from build123d import *

# Parameters (mm, degrees)
SKETCH8_R           = 12.426789642
BOSS_EXTRUDE3_DEPTH = 8.89
BOSS_EXTRUDE3_TAPER = 15
SKETCH9_R           = 9.553107684
CUT_EXTRUDE1_DEPTH  = 0.508
CUT_EXTRUDE4_REACH  = 23.683


with BuildPart() as part:
    # Sketch7 → Revolve1 (revolve)
    with BuildSketch(Plane.XY, mode=Mode.PRIVATE) as revolve1_sk:
        Polygon((9.553107684, 0), (5.743107684, 3.81), (8.616789642, 3.81), (12.426789642, 0), align=None)
    revolve(revolve1_sk.sketch.rotate(Axis((0, 0, 0), (0, 1, 0)), 90), axis=Axis((0, 0, 0), (0, 1, 0)))

    # Sketch8 → Boss-Extrude3 (add)
    with BuildSketch(Plane.XZ):
        Circle(SKETCH8_R)
    extrude(amount=BOSS_EXTRUDE3_DEPTH, taper=BOSS_EXTRUDE3_TAPER)

    # Sketch9 → Cut-Extrude1 (cut)
    with BuildSketch(Plane(origin=(0, 0, 0), x_dir=(1, 0, 0), z_dir=(0, 1, 0))):
        with Locations(Location((0, 0, 0), (0, 0, 270))):
            Circle(SKETCH9_R)
    extrude(amount=-CUT_EXTRUDE1_DEPTH, mode=Mode.SUBTRACT)

    # Cut-Extrude4: up to this face of the body (flat: up to its plane)
    cut_extrude4_end = Plane(part.part.faces().sort_by_distance((0, -0.508, 0))[0])
    # Sketch13 → Cut-Extrude4 (cut, up to the picked face)
    with BuildSketch(Plane(origin=(0, 3.81, 0), x_dir=(1, 0, 0), z_dir=(0, 1, 0)), mode=Mode.PRIVATE) as cut_extrude4_sk1:
        with BuildLine():
            Line((-5.743107684, 0), (-8.89978102, 8.672888712))
            ThreePointArc((-8.89978102, 8.672888712), (0, 12.426789642), (8.89978102, 8.672888712))
            Line((8.89978102, 8.672888712), (5.743107684, 0))
            ThreePointArc((5.743107684, 0), (0, 5.743107684), (-5.743107684, 0))
        make_face()
    cut_extrude4_tool1 = split(extrude(cut_extrude4_sk1.sketch, amount=-CUT_EXTRUDE4_REACH, mode=Mode.PRIVATE), bisect_by=cut_extrude4_end, keep=Keep.BOTH, mode=Mode.PRIVATE)
    add(cut_extrude4_tool1.solids().sort_by(Axis((0, 3.81, -7.700849), (0, -1, 0)))[0], mode=Mode.SUBTRACT)


solid = part.part
Can you work these out from the model? Positions are in its coordinate system, mm. A direction names the side the tool comes from. Round coordinates to 2 decimals unless told otherwise and drop trailing zeros. Write each loop counter-clockwise with the first axis right and the second up, starting at its lowest first coordinate (ties: lowest second). Pieces come first, ordered by that corner, then holes. Notation, with made-up numbers: M 86.5,38.5 L 141.5,38.5 A27 ccw 141.5,71.5 Z; hole C 5.5,-12.75 d10. An arc over 180 degrees is marked long. Use a Markdown table: item, result.
Item 1: I want a section at B-B (y = -5). List the corners of the cut face in (x, z) for me, and give its area (3 significant figures).
Found:
| item | result |
|---|---|
| outline | C 0,0 d22.17 |
| area | 386 mm2 |
Item 2: I want a section at D-D (y = 1). List the corners of the cut face in (x, z) for me.
Found:
| item | result |
|---|---|
| outline | M -8.52,-7.62 L -7.34,-4.39 A8.55 cw long 7.34,-4.39 L 8.52,-7.62 A11.43 ccw long Z |
Item 3: If I drill on line 1 along Y through (x, z) = (-3.75, -1.25); line 2 along Y through (x, z) = (6.75, 6.5); line 3 along X through (y, z) = (-0.15, 0), over which ranges is the centre line in solid material (lowest first)? Write a range as [from, to].
Found:
| item | result |
|---|---|
| line 1 | y = [-8.89, -0.51] |
| line 2 | y = [-8.89, -0.51], [0.18, 3.06] |
| line 3 | x = [-12.39, -9.55], [9.55, 12.39] |
Item 4: I want a section at A-A (x = 0). List the corners of the cut face in (y, z) for me.
Found:
| item | result |
|---|---|
| outline | M -8.89,-10.04 L -0.51,-12.29 L -0.51,9.55 L 0,9.55 L 3.81,5.74 L 3.81,8.62 L 0,12.43 L -8.89,10.04 Z |
Item 5: We'd pull the mould along Z, two halves only. Please class faces 3 (the face through (-0.29, 3.57, 8.85)), 4 (the face through (-0.182, 3.625, 5.925)), 5 (the face through (0, -8.89, 0)), 6 (the face through (-0.29, -0.25, 9.55)): released by +Z, released by -Z, zero draft, split by the parting line, or undercut.
Found:
| item | result |
|---|---|
| face 3 | split by the parting line |
| face 4 | undercut |
| face 5 | zero draft |
| face 6 | undercut |
Item 6: For pin 1 Ø5.5 at (x, z) = (0.5, -0.5) entering from +Y; pin 2 Ø1 at (x, z) = (8.5, 6.5) entering from +Y; pin 3 Ø6 at (y, z) = (-2, 8) entering from -X, each with a flat end and sliding along its axis, tell me the tip position at first contact or that it passes through.
Found:
| item | result |
|---|---|
| pin 1 | stops at y = -0.51 |
| pin 2 | stops at y = 2.23 |
| pin 3 | stops at x = -11.04 |
Item 7: I want a section at C-C (y = -2.5). List the corners of the cut face in (x, z) for me, and give its area (3 significant figures).
Found:
| item | result |
|---|---|
| outline | C 0,0 d23.51 |
| area | 434 mm2 |
Item 8: Which directions (+Z, -Z, +X, -X, +Y, -Y) give clear straight access to the entire face, cutting with the end or side of a thin tool? Please do faces 1 (the face through (9.944, -7.471, 3.131)), 2 (the face through (7.694, 1.681, -5.361)).
Found:
| item | result |
|---|---|
| face 1 | -Y |
| face 2 | -Z, +Y |
